```python
from build123d import *

# Parameters (mm, degrees)
SZKIC1_W        = 570
SZKIC1_H        = 5
ZAOKR_GLENIE1_R = 2


with BuildPart() as part:
    # Szkic1 → Obrót1 (revolve)
    with BuildSketch(Plane.XY, mode=Mode.PRIVATE) as obr_t1_sk:
        with Locations((126.315789474, 72.5)):
            Rectangle(SZKIC1_W, SZKIC1_H)
    revolve(obr_t1_sk.sketch.rotate(Axis((0, 0, 0), (1, 0, 0)), 90), axis=Axis((0, 0, 0), (1, 0, 0)))

    # Zaokrąglenie1
    zaokr_glenie1_edges = [part.edges().sort_by_distance(p)[0] for p in [
        (-158.684210526, 0, -75),
        (411.315789474, 0, -75),
        (411.315789474, 0, -70),
        (-158.684210526, 0, -70),
    ]]
    fillet(zaokr_glenie1_edges, radius=ZAOKR_GLENIE1_R)


solid = part.part
```
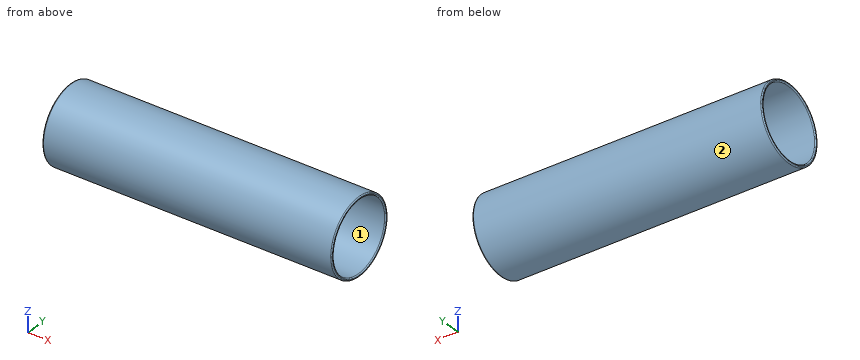
Geometry check sheet. Reference: the model listing, model coordinates, mm. Face numbers are marked on the shaded views. Coordinates: 2 decimals unless noted, no trailing zeros. Write each loop counter-clockwise with the first axis right and the second up, starting at its lowest first coordinate (ties: lowest second). Pieces come first, ordered by that corner, then holes. Notation, with made-up numbers: M -36.75,10.5 L -6.75,10.5 A26 cw -6.75,32.5 Z; hole C 31.25,81 d10. An arc over 180 degrees is marked long. Answer as a JSON object with one key per item and string values.
1. Section check A-A, the plane y = 0. Enter the section's corners in (x, z), plus the area to 3 significant figures.
Answers below:
{"outline": "M -158.68,-73 A2 ccw -156.68,-75 L 409.32,-75 A2 ccw 411.32,-73 L 411.32,-72 A2 ccw 409.32,-70 L -156.68,-70 A2 ccw -158.68,-72 Z; M -158.68,72 A2 ccw -156.68,70 L 409.32,70 A2 ccw 411.32,72 L 411.32,73 A2 ccw 409.32,75 L -156.68,75 A2 ccw -158.68,73 Z", "area": "5,690 mm²"}
2. Section check C-C, the plane x = -73.5. Enter the section's corners in (y, z).
Answers below:
{"outline": "C 0,0 d150; hole C 0,0 d140"}
3. Draft check along Y on the marked faces 1 and 2. Enter one of: released by +Y, released by -Y, zero draft, split by the parting line, or undercut.
Answers below:
{"face 1": "undercut", "face 2": "split by the parting line"}
4. Go/stop test with flat-tipped pins: pin 1 Ø1.5 at (x, z) = (346.5, 23.5) entering from +Y; pin 2 Ø5 at (x, y) = (140, 34) entering from -Z; pin 3 Ø12 at (x, z) = (44, 44.5) entering from +Y. Record where each tip stops, or that it passes through.
Answers below:
{"pin 1": "stops at y = 71.47", "pin 2": "stops at z = -68.06", "pin 3": "stops at y = 64.36"}
5. Scan lines: L1, parallel to Y at x = 13.5, z = 0; L2, parallel to Z at x = 218, y = -16; L3, parallel to Y at x = 131.5, z = -19. Record each from-to range of solid material in increasing order.
Answers below:
{"L1": "y = -75 to -70, 70 to 75", "L2": "z = -73.27 to -68.15, 68.15 to 73.27", "L3": "y = -72.55 to -67.37, 67.37 to 72.55"}
